Verification items for this drawing (mm, ordinates from the low corner). Round coordinates to 2 decimals unless told otherwise and drop trailing zeros. Order: outer loops, then holes, each group sorted by start corner. A loop starts at its lowest first (then second) coordinate and runs counter-clockwise, first axis right, second up.
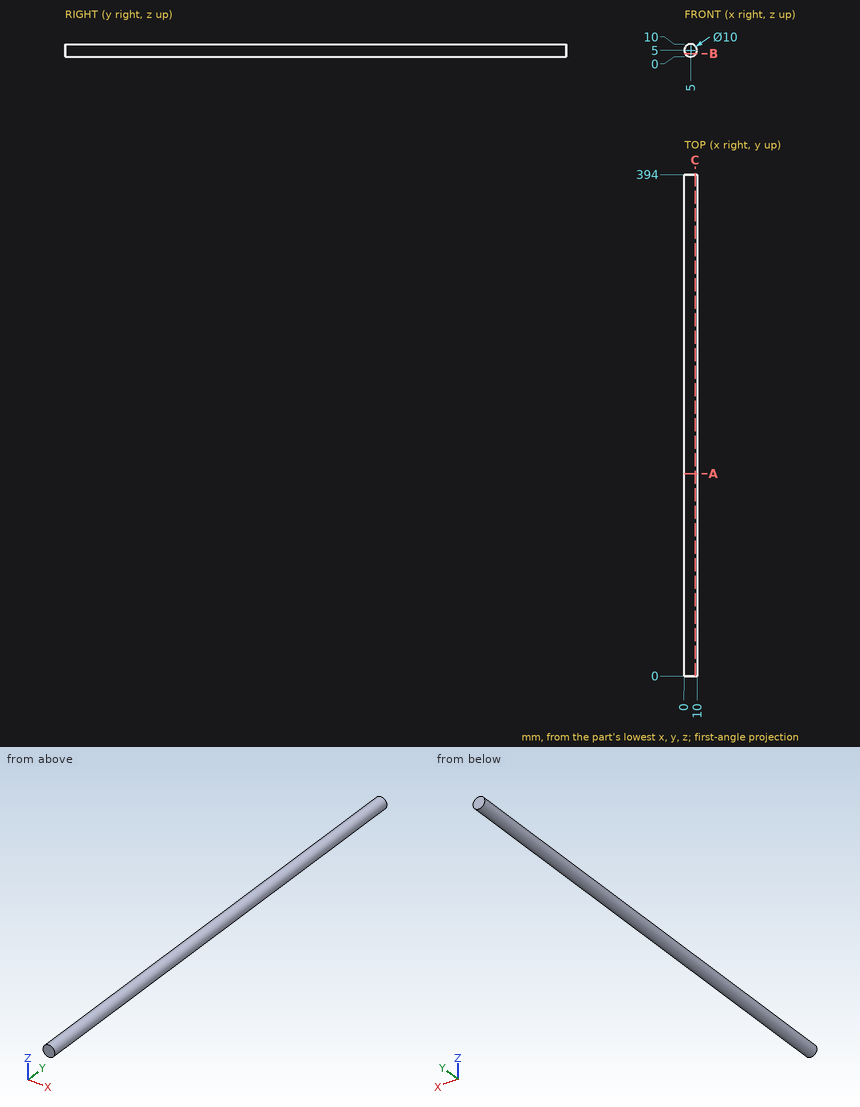
Item 1: Sectioned sample at A-A (y = 159). Record the cut outline in (x, z), and give its area (3 significant figures).
Answer:
outline: circle Ø10 at (5, 5)
area: 78.5 mm2
Item 2: Scan lines: line 1 along Z through (x, y) = (4.75, 340); line 2 along X through (y, z) = (131, 5.75); line 3 along X through (y, z) = (69, 1.5). Record each from-to range of solid material in increasing order.
Answer:
line 1: z = 0.01 to 9.99
line 2: x = 0.06 to 9.94
line 3: x = 1.43 to 8.57
Item 3: Sectioned sample at C-C (x = 8.5). Record the cut outline in (y, z).
Answer:
outline: (0, 1.43) - (394, 1.43) - (394, 8.57) - (0, 8.57) - close
Item 4: Go/stop test with flat-tipped pins: P1, Ø3, axis at y = 251, z = 2.5, coming from the +X side; P2, Ø1, axis at x = 8.5, y = 158, coming from the -Z side; P3, Ø4, axis at x = 2, y = 306, coming from the -Z side. Record where each tip stops, or that it passes through.
Answer:
P1: stops at x = 9.9
P2: stops at z = 1
P3: stops at z = 0.1
Item 5: Sectioned sample at B-B (z = 2.5). Record the cut outline in (x, y), and give its area (3 significant figures).
Answer:
outline: (0.67, 0) - (9.33, 0) - (9.33, 394) - (0.67, 394) - close
area: 3,410 mm2
